```python
from build123d import *

# Parameters (mm, degrees)
PAD_DEPTH = 40


with BuildPart() as part:
    # Sketch → Pad (new body)
    with BuildSketch(Plane.XZ):
        with BuildLine():
            Line((0, 0), (120, 0))
            Line((120, 0), (120, 58.867513))
            ThreePointArc((120, 58.867513), (114.142136, 73.009649), (100, 78.867513))
            Line((50, 78.867513), (100, 78.867513))
            Line((0, 50), (50, 78.867513))
            Line((0, 0), (0, 50))
        make_face()
    extrude(amount=-PAD_DEPTH)


solid = part.part
```
Could you check a few things on this model? Use its own coordinates, in mm. Round coordinates to 2 decimals unless told otherwise and drop trailing zeros. Loops run counter-clockwise (first coordinate to the right, second up) from the corner with the lowest first, then second, coordinate; pieces in that order, holes last. Notation, with made-up numbers: (82, 86.5) - (135, 86.5) arc R19 ccw to (135, 92.5) - close; hole circle Ø10 at (-15.5, 24). An arc over 180 degrees is marked (long way). Answer in a Markdown table with one row per item. Add a question column.
(1) I need wall thicknesses on line 1 along Z through (x, y) = (44, 14); line 2 along Z through (x, y) = (22, 16); line 3 along X through (y, z) = (22.5, 57.5). Which ranges of each line are inside material? Lowest first, please.
(2) If we section it at C-C (x = 109.5): Please give me the cut outline in (y, z), plus the area to 3 significant figures.
(3) If we section it at B-B (z = 53): Please give me the cut outline in (x, y), plus the area to 3 significant figures.
(4) If we section it at A-A (y = 3): Please give me the cut outline in (x, z), plus the area to 3 significant figures.
Model answer:
| question | item | result |
|---|---|---|
| 1 | line 1 | z = 0 to 75.4 |
| 1 | line 2 | z = 0 to 62.7 |
| 1 | line 3 | x = 12.99 to 120 |
| 2 | outline | (0, 0) - (40, 0) - (40, 76.47) - (0, 76.47) - close |
| 2 | area | 3,060 mm² |
| 3 | outline | (5.2, 0) - (120, 0) - (120, 40) - (5.2, 40) - close |
| 3 | area | 4,590 mm² |
| 4 | outline | (0, 0) - (120, 0) - (120, 58.87) arc R20 ccw to (100, 78.87) - (50, 78.87) - (0, 50) - close |
| 4 | area | 8,660 mm² |
